Source: CAD feature listing. Evaluate the final solid. Frame: model axes, mm. A direction names the side the tool comes from. Round coordinates to 2 decimals unless told otherwise and drop trailing zeros. Loops run counter-clockwise (first coordinate to the right, second up) from the corner with the lowest first, then second, coordinate; pieces in that order, holes last. Notation, with made-up numbers: M -32.5,80 L -9.5,80 A21 ccw -9.5,86 Z; hole C 38,-3 d6. An arc over 180 degrees is marked long. Write each question's results on one line, items separated by ' | '. Start each with the question number.
1. Section A-A on z = 21. Output: boundary loops of the cut face in (x, y), and give its area (3 significant figures).
2. Section B-B on y = 29.5. Output: boundary loops of the cut face in (x, z).
3. Contact query for flat-ended pins moving along their axis: pin 1 Ø16 at (x, z) = (25, 34.5) entering from -Y; pin 2 Ø6 at (y, z) = (22.5, 40.5) entering from +X; pin 3 Ø2 at (x, y) = (27.5, 36.5) entering from -Z; pin 4 Ø8 at (x, z) = (29.5, 49.5) entering from -Y. Output: stop coordinate, or through.
4. Set-up query: faces 1 (the flat face through (28, 45, 35)), 2 (the flat face through (38, 20, 50)), 3 (the flat face through (10, 40, 50)). Return all of +Z, -Z, +X, -X, +Y, -Y with unobstructed straight access to the full face (end or side cutting, diameter ignored); none if empty.
5. Ray query, line 1 (Z direction, x = 40, y = 43.5); line 2 (Y direction, x = 12, z = 11); line 3 (Y direction, x = 21, z = 41). Return the intervals inside material, ascending.
6. Section C-C on x = 6. Output: boundary loops of the cut face in (y, z), and give its area (3 significant figures).
7. Draft query along X for faces 4 (the flat face through (12, 40, 13)), 5 (the flat face through (20, 30, 50)), 6 (the flat face through (34, 33, 45)). Return one class per face: released by +X, released by -X, zero draft, split by the parting line, or undercut.
8. Section D-D on z = 49. Output: boundary loops of the cut face in (x, y).
from build123d import *

# Parameters (mm, degrees)
F0_W     = 55
F0_H     = 60
F1_DEPTH = 55
F3_DEPTH = 55.001
F4_R     = 10
F5_W     = 20
F5_H     = 20
F6_DEPTH = 10
F7_W     = 15
F7_H     = 15
F8_DEPTH = 25.001


with BuildPart() as f1:
    # F0 (on Top) → F1 (new body)
    with BuildSketch(Plane.XY):
        with Locations((27.5, 30)):
            Rectangle(F0_W, F0_H)
    extrude(amount=F1_DEPTH)

    # F2 (on face) → F3 (cut, through all)
    with BuildSketch(Plane.YZ.offset(55)):
        Polygon((20, 55), (0, 55), (0, 25), (45, 25), (45, 45), (20, 45), align=None)
    extrude(amount=-F3_DEPTH, mode=Mode.SUBTRACT)

    # F4
    f4_edges = [f1.edges().sort_by_distance(p)[0] for p in [
        (0, 60, 27.5),
    ]]
    fillet(f4_edges, radius=F4_R)

    # F5 (on face) → F6 (cut, through all)
    with BuildSketch(Plane.XY.offset(55)):
        with Locations((10, 30)):
            Rectangle(F5_W, F5_H)
    extrude(amount=-F6_DEPTH, mode=Mode.SUBTRACT)

    # F7 (on face) → F8 (cut, through all)
    with BuildSketch(Plane.XY.offset(25)):
        with Locations((12.5, 32.5)):
            Rectangle(F7_W, F7_H)
    extrude(amount=-F8_DEPTH, mode=Mode.SUBTRACT)


solid = f1.part
Taken from the geometry:
1) outline: M 0,0 L 55,0 L 55,60 L 10,60 A10 ccw 0,50 Z; hole M 5,25 L 20,25 L 20,40 L 5,40 Z | area: 3,050 mm^2
2) outline: M 0,0 L 5,0 L 5,25 L 0,25 Z; M 20,0 L 55,0 L 55,25 L 20,25 Z; M 20,45 L 55,45 L 55,55 L 20,55 Z
3) pin 1: y = 45 | pin 2: through | pin 3: z = 0 | pin 4: y = 20
4) face 1: +X, -X, -Y | face 2: +Z, +X, -X, -Y | face 3: +Z, -X, -Y
5) line 1: 0 to 25, 45 to 55 | line 2: 0 to 25, 40 to 60 | line 3: 45 to 60
6) outline: M 0,0 L 25,0 L 25,25 L 0,25 Z; M 40,0 L 59.17,0 L 59.17,55 L 40,55 L 40,45 L 45,45 L 45,25 L 40,25 Z | area: 1,580 mm^2
7) face 4: undercut | face 5: released by -X | face 6: zero draft
8) outline: M 0,40 L 20,40 L 20,20 L 55,20 L 55,60 L 10,60 A10 ccw 0,50 Z
